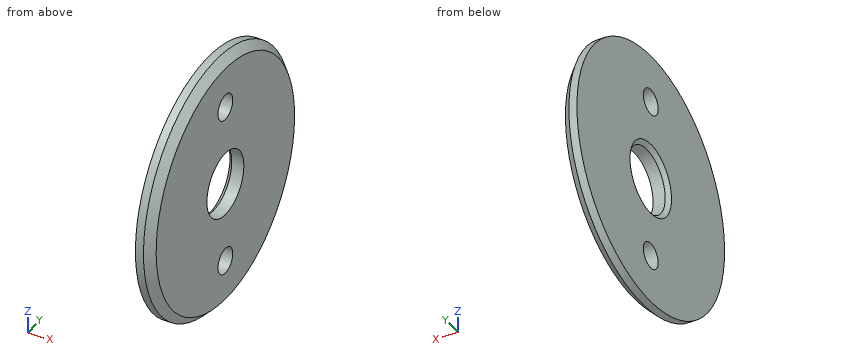
from build123d import *

# Parameters (mm, degrees)
SKETCH1_R           = 16
SKETCH1_R_2         = 4
BOSS_EXTRUDE1_DEPTH = 2
SKETCH2_R           = 1.6
CUT_EXTRUDE1_DEPTH  = 3
CHAMFER1_SIZE       = 1
CHAMFER2_SIZE       = 0.5


with BuildPart() as part:
    # Sketch1 → Boss-Extrude1 (new body)
    with BuildSketch(Plane(origin=(0, 0, 0), x_dir=(0, 0, -1), z_dir=(1, 0, 0))):
        Circle(SKETCH1_R)
        Circle(SKETCH1_R_2, mode=Mode.SUBTRACT)
    extrude(amount=BOSS_EXTRUDE1_DEPTH)

    # Sketch2 → Cut-Extrude1 (cut, through all)
    with BuildSketch(Plane(origin=(2, 0, 0), x_dir=(0, 0, -1), z_dir=(1, 0, 0))):
        with Locations((-10, 0)):
            Circle(SKETCH2_R)
        with Locations((10, 0)):
            Circle(SKETCH2_R)
    extrude(amount=-CUT_EXTRUDE1_DEPTH, mode=Mode.SUBTRACT)

    # Chamfer1
    chamfer1_edges = [part.edges().sort_by_distance(p)[0] for p in [
        (2, 0, 16),
    ]]
    chamfer(chamfer1_edges, length=CHAMFER1_SIZE)

    # Chamfer2
    chamfer2_edges = [part.edges().sort_by_distance(p)[0] for p in [
        (0, 0, 4),
    ]]
    chamfer(chamfer2_edges, length=CHAMFER2_SIZE)


solid = part.part
Build history of the part. All positions in model axes, mm. Round coordinates to 2 decimals unless told otherwise and drop trailing zeros. Write each loop counter-clockwise with the first axis right and the second up, starting at its lowest first coordinate (ties: lowest second). Pieces come first, ordered by that corner, then holes. Notation, with made-up numbers: M 45.25,67 L 98.25,67 A25 cw 98.25,79 Z; hole C 16,0.25 d3. An arc over 180 degrees is marked long. Answer as a JSON object with one key per item and string values. Group by question number.
(1) Cut at B-B (y = 0). Give the cut face in (x, z).
(2) Drill centre lines: L1, parallel to Y at x = 0.9, z = 0; L2, parallel to Z at x = 0.65, y = -3.5; L3, parallel to Z at x = 1.9, y = -2. Where is each one in solid material? Low to high.
(3) Cut at A-A (z = 0). Give the cut face in (x, y).
Responses:
{
 "1": {"outline": "M 0,-16 L 1,-16 L 2,-15 L 2,-11.6 L 0,-11.6 Z; M 0,-8.4 L 2,-8.4 L 2,-4 L 0.5,-4 L 0,-4.5 Z; M 0,4.5 L 0.5,4 L 2,4 L 2,8.4 L 0,8.4 Z; M 0,11.6 L 2,11.6 L 2,15 L 1,16 L 0,16 Z"},
 "2": {"L1": "y = -16 to -4, 4 to 16", "L2": "z = -15.61 to -1.94, 1.94 to 15.61", "L3": "z = -14.97 to -3.46, 3.46 to 14.97"},
 "3": {"outline": "M 0,-16 L 1,-16 L 2,-15 L 2,-4 L 0.5,-4 L 0,-4.5 Z; M 0,4.5 L 0.5,4 L 2,4 L 2,15 L 1,16 L 0,16 Z"}
}
